Job drawing, mm, ordinate dimensions from the low corner. One solid piece. Give positions to 0.01 mm unless a question says otherwise; leave off trailing zeros. Loops run counter-clockwise (first coordinate to the right, second up) from the corner with the lowest first, then second, coordinate; pieces in that order, holes last. Notation, with made-up numbers: M 1.25,69 L 26.25,69 A5 cw 26.25,73 Z; hole C 78.5,86.5 d9. An arc over 180 degrees is marked long. One line per question, with ' | ' between items.
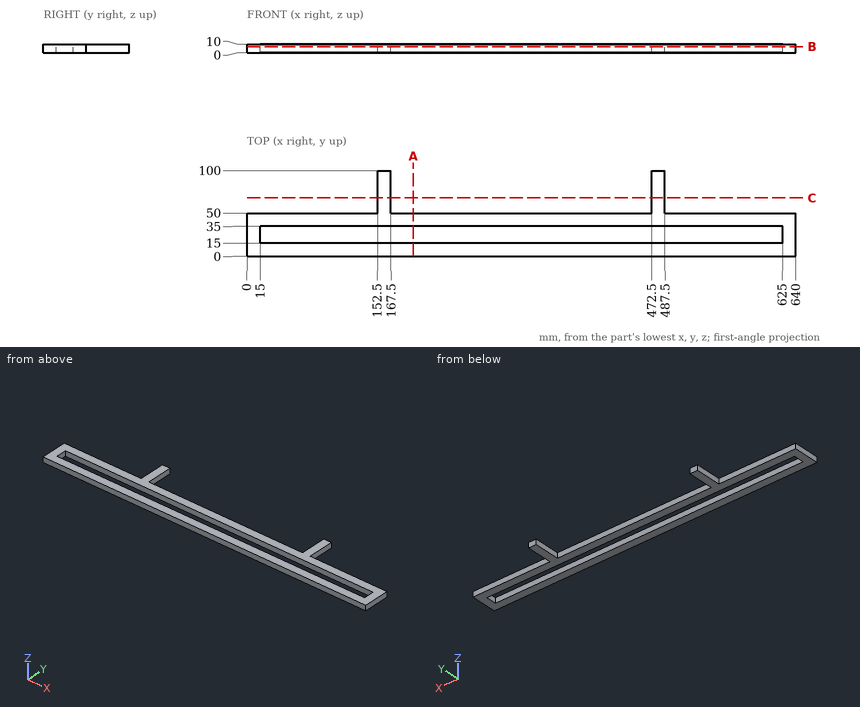
Item 1: Saw through at A-A on x = 194. Give the cut face in (y, z).
Conclusion:
outline: M 0,0 L 15,0 L 15,10 L 0,10 Z; M 35,0 L 50,0 L 50,10 L 35,10 Z
Item 2: Drop flat-ended pins along their axis: P1, Ø3, axis at x = 326, z = 3, coming from the +Y side; P2, Ø5, axis at y = 74.5, z = 7.5, coming from the -X side; P3, Ø3, axis at y = 76.5, z = 5.5, coming from the +X side. Give the stop position or say it passes through.
Conclusion:
P1: y = 50 | P2: x = 152.5 | P3: x = 487.5
Item 3: Saw through at B-B on z = 7. Give the cut face in (x, y), and give its area (3 significant figures).
Conclusion:
outline: M 0,0 L 640,0 L 640,50 L 487.5,50 L 487.5,100 L 472.5,100 L 472.5,50 L 167.5,50 L 167.5,100 L 152.5,100 L 152.5,50 L 0,50 Z; hole M 15,15 L 625,15 L 625,35 L 15,35 Z | area: 21,300 mm²
Item 4: Saw through at C-C on y = 68. Give the cut face in (x, z).
Conclusion:
outline: M 152.5,0 L 167.5,0 L 167.5,10 L 152.5,10 Z; M 472.5,0 L 487.5,0 L 487.5,10 L 472.5,10 Z
Item 5: Drill centre lines: line 1 along Y through (x, z) = (132, 0.5); line 2 along X through (y, z) = (59, 1.5); line 3 along X through (y, z) = (33.5, 0.5). Where is each one in solid material? Low to high. Write a range as [from, to].
Conclusion:
line 1: [0, 15], [35, 50] | line 2: [152.5, 167.5], [472.5, 487.5] | line 3: [0, 15], [625, 640]
